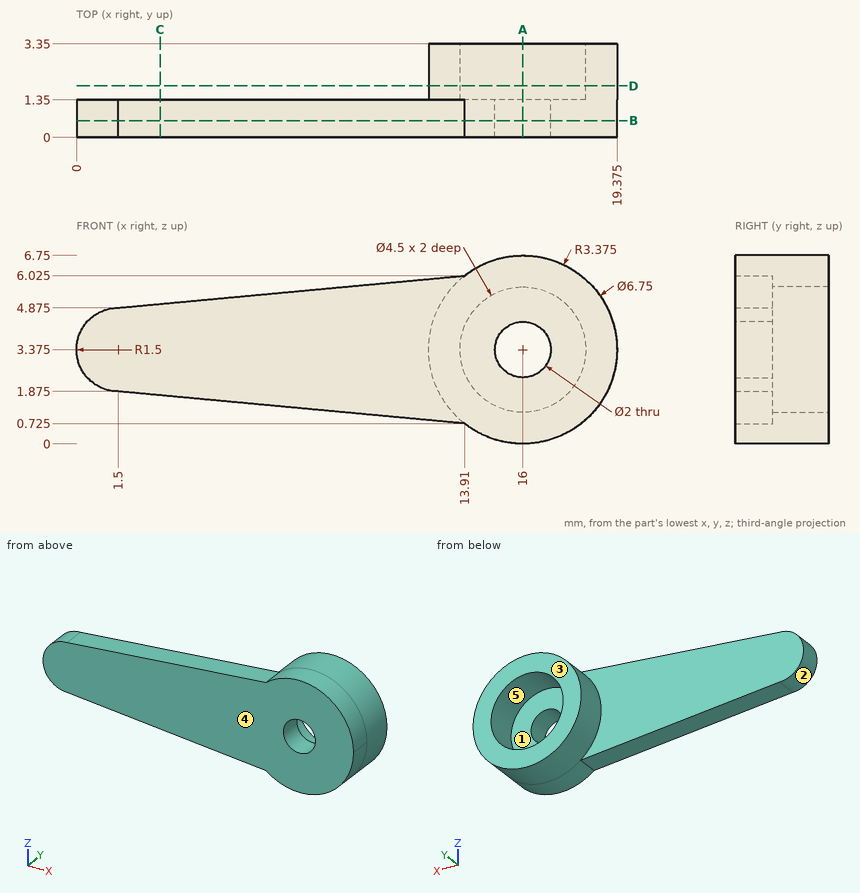
The figure shows three views and two pictorial views of one solid part (mm, origin at its lowest corner). Answer the questions. A direction names the side the tool comes from. Give positions to 0.01 mm unless a question says otherwise; leave off trailing zeros. Loops run counter-clockwise (first coordinate to the right, second up) from the corner with the lowest first, then second, coordinate; pieces in that order, holes last. Notation, with made-up numbers: (26.5, 21) -> (80.5, 21) arc R19 ccw to (80.5, 35) -> close; hole circle Ø8 at (51.25, 39.5). An arc over 180 degrees is marked (long way). Use a Markdown table: item, result. Add a question column.
1. Section B-B on y = 0.6 is taken. Determine the outline of the cut face in (x, z) (3 decimals).
2. A flat-ended cylindrical pin translates along its axis: pin 1 Ø1.6 at (x, z) = (10, 2.5) entering from +Y. Find the tip coordinate at first contact, or state that the pin passes through.
3. For the marked faces 4 and 5, determine the directions among +Z, -Z, +X, -X, +Y, -Y from which every point of the face is accessible in a straight line to the end or side of a thin tool.
4. Find the intervals of material crossed by probe 1 along Y at (x, z) = (6.5, 3); probe 2 along X at (y, z) = (1.6, 3.75); probe 3 along X at (y, z) = (0.55, 3.5), in increasing order.
5. Section C-C on x = 3 is taken. Determine the outline of the cut face in (y, z).
6. Section A-A on x = 16 is taken. Determine the outline of the cut face in (y, z) (3 decimals).
7. Section D-D on y = 1.85 is taken. Determine the outline of the cut face in (x, z) (3 decimals), and give its area (3 significant figures).
8. Determine the mould class of the marked faces 1, 2 and 3 for opening direction Z: released by +Z, released by -Z, zero draft, split by the parting line, or undercut.
Results below:
| question | item | result |
|---|---|---|
| 1 | outline | (1.5, 1.875) -> (13.91, 0.725) arc R3.375 ccw (long way) to (13.91, 6.025) -> (1.5, 4.875) arc R1.5 ccw to start; hole circle Ø2 at (16, 3.375) |
| 2 | pin 1 | stops at y = 1.35 |
| 3 | face 4 | +Z, -Z, +X, -X, -Y |
| 3 | face 5 | +Y |
| 4 | probe 1 | y = 0 to 1.35 |
| 4 | probe 2 | x = 12.65 to 13.78, 18.22 to 19.35 |
| 4 | probe 3 | x = 0.01 to 15.01, 16.99 to 19.37 |
| 5 | outline | (0, 1.74) -> (1.35, 1.74) -> (1.35, 5.01) -> (0, 5.01) -> close |
| 6 | outline | (0, 0) -> (3.35, 0) -> (3.35, 1.125) -> (1.35, 1.125) -> (1.35, 2.375) -> (0, 2.375) -> close; (0, 4.375) -> (1.35, 4.375) -> (1.35, 5.625) -> (3.35, 5.625) -> (3.35, 6.75) -> (0, 6.75) -> close |
| 7 | outline | circle Ø6.75 at (16, 3.375); hole circle Ø4.5 at (16, 3.375) |
| 7 | area | 19.9 mm^2 |
| 8 | face 1 | undercut |
| 8 | face 2 | split by the parting line |
| 8 | face 3 | zero draft |
